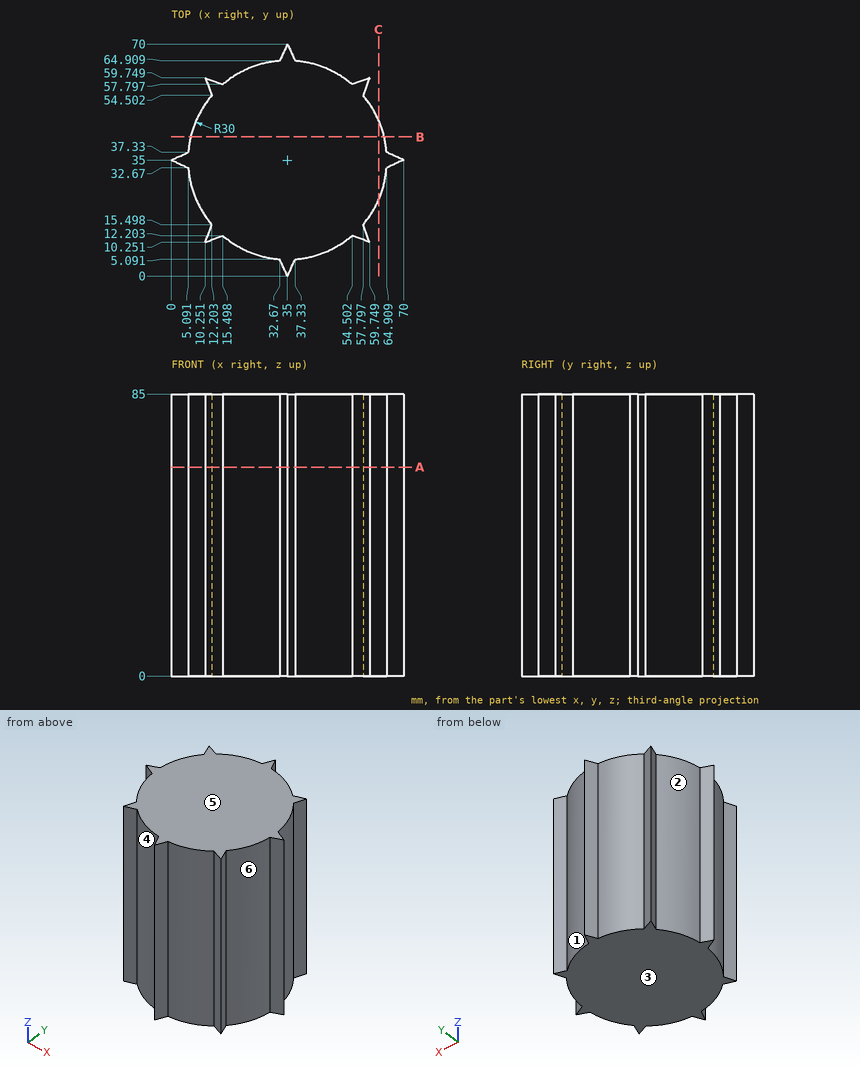
Source: three-view drawing plus pictorial views. Frame: mm from the lowest corner of the part. A direction names the side the tool comes from. Coordinates: 2 decimals unless noted, no trailing zeros. Loops run counter-clockwise (first coordinate to the right, second up) from the corner with the lowest first, then second, coordinate; pieces in that order, holes last. Notation, with made-up numbers: M 74,31 L 104,31 A30 ccw 104,64 Z; hole C 62.25,14 d9. An arc over 180 degrees is marked long. Use CSV: the item, a comma, the result in double quotes.
(1) Cut plane B-B on y = 42. Return loops of the section in (x, z).
Answers follow:
outline,"M 5.83,0 L 64.17,0 L 64.17,85 L 5.83,85 Z"
(2) Cut plane C-C on x = 62.5. Return loops of the section in (y, z).
Answers follow:
outline,"M 23.01,0 L 46.99,0 L 46.99,85 L 23.01,85 Z"
(3) Cut plane A-A on z = 63. Return loops of the section in (x, y), and give its area (3 significant figures).
Answers follow:
outline,"M 0,35 L 5.09,32.67 A30 ccw 12.2,15.5 L 10.25,10.25 L 15.5,12.2 A30 ccw 32.67,5.09 L 35,0 L 37.33,5.09 A30 ccw 54.5,12.2 L 59.75,10.25 L 57.8,15.5 A30 ccw 64.91,32.67 L 70,35 L 64.91,37.33 A30 ccw 57.8,54.5 L 59.75,59.75 L 54.5,57.8 A30 ccw 37.33,64.91 L 35,70 L 32.67,64.91 A30 ccw 15.5,57.8 L 10.25,59.75 L 12.2,54.5 A30 ccw 5.09,37.33 Z"
area,"2,920 mm²"
(4) Contact query for flat-ended pins moving along their axis: pin 1 (1.5 mm diameter, centred on x = 8.5, z = 73, fed in from +Y) (1 decimal); pin 2 (4 mm diameter, centred on x = 14, z = 73, fed in from -Y); pin 3 (1 mm diameter, centred on y = 19.5, z = 73, fed in from -X). Output: stop coordinate, or through.
Answers follow:
pin 1,"y = 50.4"
pin 2,"y = 10.9"
pin 3,"x = 9.02"
(5) Reachability of the marked faces 1, 2 and 3 from +Z, -Z, +X, -X, +Y, -Y: full face, straight path, thin tool, end or side. Return the list, or none.
Answers follow:
face 1,"+Z, -Z, +Y"
face 2,"+Z, -Z, -X"
face 3,"-Z, +X, -X, +Y, -Y"
(6) Draft query along X for the marked faces 4, 5 and 6. Return one class per face: pulls with the +X half, pulls with the -X half, needs draft (parallel to the pull), parting line crosses it, or undercut.
Answers follow:
face 4,"undercut"
face 5,"needs draft"
face 6,"pulls with the +X half"
(7) Line query: line 1 (Y direction, x = 4, z = 51.5); line 2 (X direction, y = 16, z = 50) (1 decimal); line 3 (X direction, y = 44, z = 73.5). Output: solid intervals per line, ascending. Write a range as [from, to].
Answers follow:
line 1,"[33.17, 36.83]"
line 2,"[11.8, 58.2]"
line 3,"[6.38, 63.62]"
